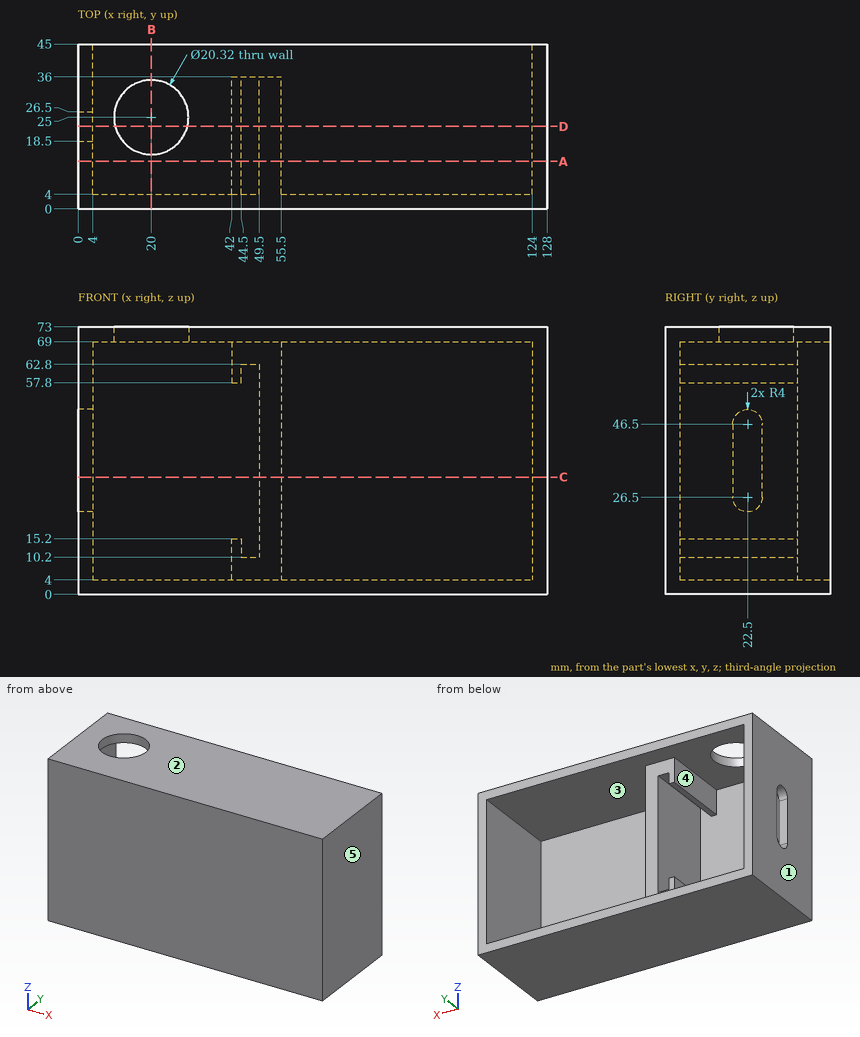
Study the drawing (mm; zero at the part's minimum x, y, z) and answer. A direction names the side the tool comes from. Round coordinates to 2 decimals unless told otherwise and drop trailing zeros. Loops run counter-clockwise (first coordinate to the right, second up) from the corner with the lowest first, then second, coordinate; pieces in that order, holes last.
Q1. Section C-C, the plane z = 32 is taken. Determine the outline of the cut face in (x, y), then the cut area to 3 significant figures.
Q2. Which of the six approach directions +Z, -Z, +X, -X, +Y, -Y give full straight-line access (tool end or side, diameter ignored) to the marked faces 4 and 5?
Q3. Find the intervals of material crossed by line 1 (X direction, y = 34, z = 55.5); line 2 (X direction, y = 20, z = 66); line 3 (Y direction, x = 20, z = 71), in increasing order.
Q4. Section A-A, the plane y = 13 is taken. Determine the outline of the cut face in (x, z), then the cut area to 3 significant figures.
Q5. Section B-B, the plane x = 20 is taken. Determine the outline of the cut face in (y, z).
Q6. For a pull along Z with two mould halves and no side action, classify the marked faces 1, 2 and 3 as released by +Z, released by -Z, zero draft, split by the parting line, or undercut.
Q7. Section D-D, the plane y = 22.5 is taken. Determine the outline of the cut face in (x, z).
Q8. Given pin 1 Ø1 at (y, z) = (21, 27) entering from -X; pin 2 Ø4 at (x, z) = (52, 52) entering from +Y, each flat-ended and moving along its own axis, determine where each tip first touches the part or whether it passes through.
Completed:
1. outline: (0, 0) - (128, 0) - (128, 45) - (124, 45) - (124, 4) - (55.5, 4) - (55.5, 36) - (49.5, 36) - (49.5, 4) - (4, 4) - (4, 18.5) - (0, 18.5) - close; (0, 26.5) - (4, 26.5) - (4, 45) - (0, 45) - close
1. area: 1,000 mm2
2. face 4: +Y
2. face 5: +Z, -Z, +X, +Y, -Y
3. line 1: x = 0 to 4, 49.5 to 55.5, 124 to 128
3. line 2: x = 0 to 4, 42 to 55.5, 124 to 128
3. line 3: y = 0 to 14.84, 35.16 to 45
4. outline: (0, 0) - (128, 0) - (128, 73) - (0, 73) - close; hole (4, 4) - (42, 4) - (42, 15.2) - (44.5, 15.2) - (44.5, 10.2) - (49.5, 10.2) - (49.5, 62.8) - (44.5, 62.8) - (44.5, 57.8) - (42, 57.8) - (42, 69) - (4, 69) - close; hole (55.5, 4) - (124, 4) - (124, 69) - (55.5, 69) - close
4. area: 2,050 mm2
5. outline: (0, 0) - (45, 0) - (45, 4) - (4, 4) - (4, 69) - (14.84, 69) - (14.84, 73) - (0, 73) - close; (35.16, 69) - (45, 69) - (45, 73) - (35.16, 73) - close
6. face 1: zero draft
6. face 2: released by +Z
6. face 3: undercut
7. outline: (0, 0) - (128, 0) - (128, 73) - (29.85, 73) - (29.85, 69) - (42, 69) - (42, 57.8) - (44.5, 57.8) - (44.5, 62.8) - (49.5, 62.8) - (49.5, 10.2) - (44.5, 10.2) - (44.5, 15.2) - (42, 15.2) - (42, 4) - (4, 4) - (4, 22.5) - (0, 22.5) - close; (0, 50.5) - (4, 50.5) - (4, 69) - (10.15, 69) - (10.15, 73) - (0, 73) - close; hole (55.5, 4) - (124, 4) - (124, 69) - (55.5, 69) - close
8. pin 1: stops at x = 49.5
8. pin 2: stops at y = 36
